Input: dimensioned drawing with shaded views. Units: mm. Origin: part minimum x, y, z. Coordinates: 2 decimals unless noted, no trailing zeros. Loops run counter-clockwise (first coordinate to the right, second up) from the corner with the lowest first, then second, coordinate; pieces in that order, holes last. Notation, with made-up numbers: (71.5, -4.75) - (79.5, -4.75) arc R22 ccw to (79.5, 31.25) - close; hole circle Ø10 at (-36.75, 36.5). An arc over 180 degrees is marked (long way). Put each result on its own line as item: value. Start each with the question number.
1) Section B-B on x = 58. Output: boundary loops of the cut face in (y, z).
2) Material intervals for line 1 along Y through (x, z) = (15, 2.2); line 2 along Y through (x, z) = (58, 2.3); line 3 along X through (y, z) = (86.5, 4.2), sorted ascending. Write a range as from..to.
3) Section A-A on y = 83. Output: boundary loops of the cut face in (x, z).
4) Section C-C on x = 101. Output: boundary loops of the cut face in (y, z), and give its area (3 significant figures).
5) Section D-D on z = 3.15. Output: boundary loops of the cut face in (x, y).
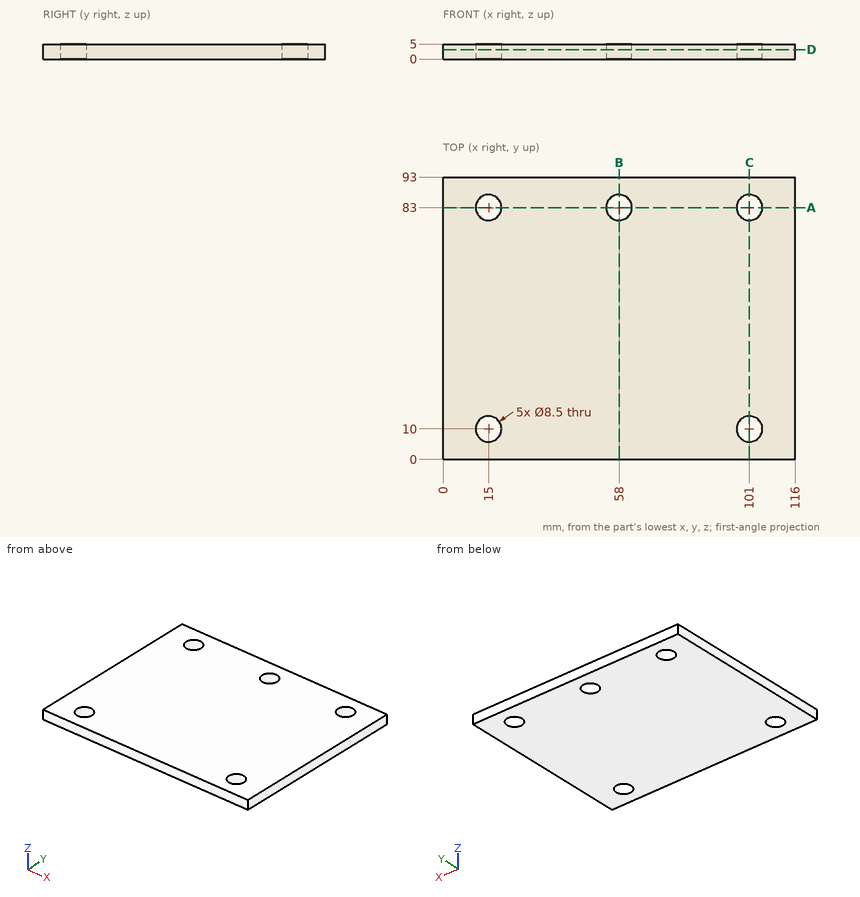
Answer block:
1. outline: (0, 0) - (78.75, 0) - (78.75, 5) - (0, 5) - close; (87.25, 0) - (93, 0) - (93, 5) - (87.25, 5) - close
2. line 1: y = 0..5.75, 14.25..78.75, 87.25..93
2. line 2: y = 0..78.75, 87.25..93
2. line 3: x = 0..12.59, 17.41..55.59, 60.41..98.59, 103.41..116
3. outline: (0, 0) - (10.75, 0) - (10.75, 5) - (0, 5) - close; (19.25, 0) - (53.75, 0) - (53.75, 5) - (19.25, 5) - close; (62.25, 0) - (96.75, 0) - (96.75, 5) - (62.25, 5) - close; (105.25, 0) - (116, 0) - (116, 5) - (105.25, 5) - close
4. outline: (0, 0) - (5.75, 0) - (5.75, 5) - (0, 5) - close; (14.25, 0) - (78.75, 0) - (78.75, 5) - (14.25, 5) - close; (87.25, 0) - (93, 0) - (93, 5) - (87.25, 5) - close
4. area: 380 mm²
5. outline: (0, 0) - (116, 0) - (116, 93) - (0, 93) - close; hole circle Ø8.5 at (15, 10); hole circle Ø8.5 at (15, 83); hole circle Ø8.5 at (58, 83); hole circle Ø8.5 at (101, 10); hole circle Ø8.5 at (101, 83)
